Here's the drawing with two shaded views (mm, measured from the low corner). I have some questions. Round coordinates to 2 decimals unless told otherwise and drop trailing zeros. Loops run counter-clockwise (first coordinate to the right, second up) from the corner with the lowest first, then second, coordinate; pieces in that order, holes last.
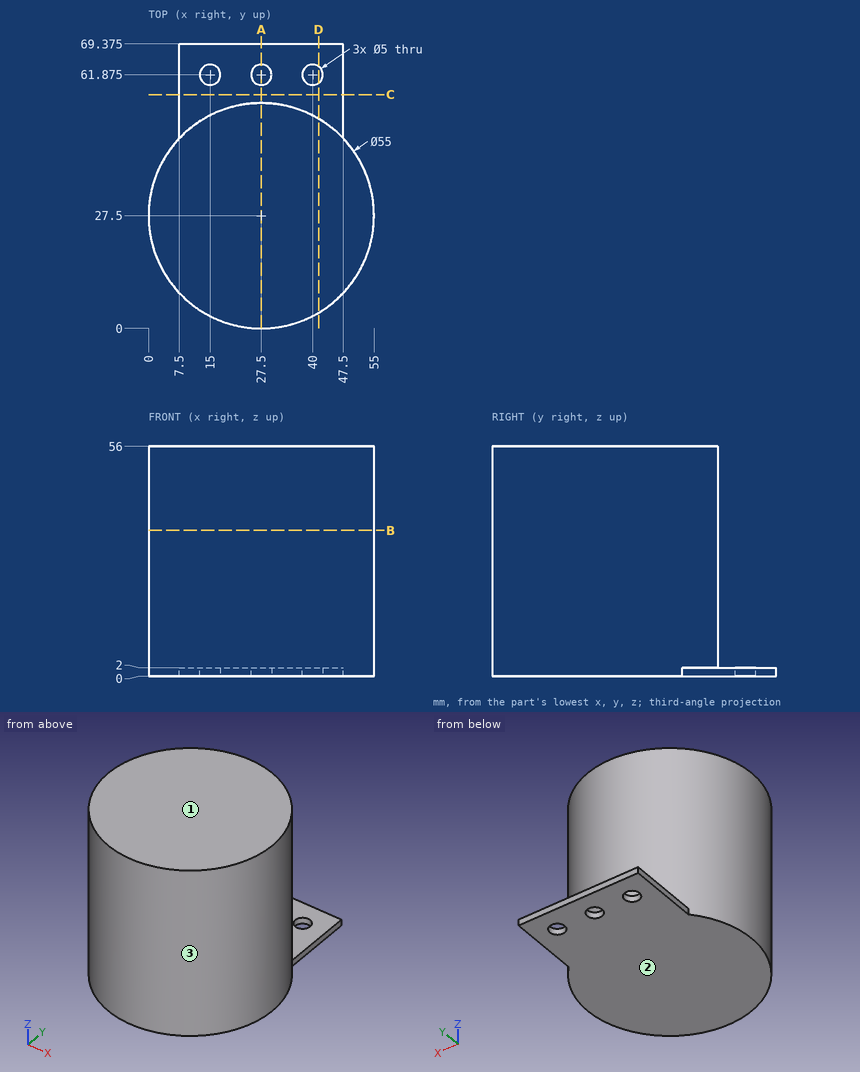
Item 1: We'd pull the mould along Z, two halves only. Please class the marked faces 1, 2 and 3: released by +Z, released by -Z, zero draft, split by the parting line, or undercut.
Results list:
face 1: released by +Z
face 2: released by -Z
face 3: zero draft
Item 2: If we section it at A-A, the plane x = 27.5: Please give me the cut outline in (y, z) (1 decimal).
Results list:
outline: (0, 0) - (59.4, 0) - (59.4, 2) - (55, 2) - (55, 56) - (0, 56) - close; (64.4, 0) - (69.4, 0) - (69.4, 2) - (64.4, 2) - close
Item 3: Will these pins go through, and if not, where does the flat tip stop? pin 1 (1 mm diameter, centred on x = 16, z = 38.5, fed in from +Y) (1 decimal); pin 2 (12 mm diameter, centred on y = 40, z = 35, fed in from +X); pin 3 (0.6 mm diameter, centred on y = 57, z = 0.5, fed in from -X); pin 4 (4.5 mm diameter, centred on x = 40, y = 61.87, fed in from +Z).
Results list:
pin 1: stops at y = 52.7
pin 2: stops at x = 54.22
pin 3: stops at x = 7.5
pin 4: passes through
Item 4: If we section it at B-B, the plane z = 35.5: Please give me the cut outline in (x, y), then the cut area to 3 significant figures.
Results list:
outline: circle Ø55 at (27.5, 27.5)
area: 2,380 mm2
Item 5: If we section it at C-C, the plane y = 57: Please give me the cut outline in (x, z).
Results list:
outline: (7.5, 0) - (47.5, 0) - (47.5, 2) - (7.5, 2) - close
Item 6: If I drill on line 1 along Y through (x, z) = (27.5, 0.9) (1 decimal); line 2 along Z through (x, y) = (17, 64.5); line 3 along Y through (x, z) = (40, 1) (1 decimal), over which ranges is the centre line in solid material (lowest first)?
Results list:
line 1: y = 0 to 59.4, 64.4 to 69.4
line 2: z = 0 to 2
line 3: y = 3 to 59.4, 64.4 to 69.4
Item 7: If we section it at D-D, the plane x = 41.5: Please give me the cut outline in (y, z) (1 decimal).
Results list:
outline: (3.8, 0) - (59.9, 0) - (59.9, 2) - (51.2, 2) - (51.2, 56) - (3.8, 56) - close; (63.9, 0) - (69.4, 0) - (69.4, 2) - (63.9, 2) - close
